from build123d import *

# Parameters (mm, degrees)
F0_R     = 2
F1_DEPTH = 2.5
F2_DEPTH = 4
F3_DEPTH = 8.5
F4_DEPTH = 2
F5_R     = 0.99999


# Not quite as in the source:
# - a fillet or chamfer is up to 0.001 mm smaller than in the source, because OpenCascade refuses the exact size


with BuildPart() as f1:
    # F0 (on Front) → F1 (new body)
    with BuildSketch(Plane.XZ):
        with BuildLine():
            Line((2, 3.4641016151), (2, 0))
            ThreePointArc((2, 0), (0, -2), (-2, 0))
            Line((-2, 0), (-4, 0))
            ThreePointArc((-4, 0), (-2.8284271247, -2.8284271247), (0, -4))
            ThreePointArc((0, -4), (2.8284271247, -2.8284271247), (4, 0))
            ThreePointArc((4, 0), (3.4641016151, 2), (2, 3.4641016151))
        make_face()
        with BuildLine():
            ThreePointArc((0, 4), (1.0352761804, 3.8637033052), (2, 3.4641016151))
            Line((2, 3.4641016151), (2, 4))
            Line((2, 4), (0, 4))
        make_face()
        with BuildLine():
            Line((2, 4), (2, 3.4641016151))
            ThreePointArc((2, 3.4641016151), (3.4641016151, 2), (4, 0))
            ThreePointArc((4, 0), (2.8284271247, -2.8284271247), (0, -4))
            Line((0, -4), (15.6, -4))
            ThreePointArc((15.6, -4), (19.6, 0), (15.6, 4))
            Line((15.6, 4), (2, 4))
        make_face()
        with Locations((15.6, 0)):
            Circle(F0_R, mode=Mode.SUBTRACT)
        with BuildLine():
            ThreePointArc((-2, 0), (0, 2), (2, 0))
            Line((2, 0), (2, 3.4641016151))
            ThreePointArc((2, 3.4641016151), (1.0352761804, 3.8637033052), (0, 4))
            ThreePointArc((0, 4), (-2.8284271247, 2.8284271247), (-4, 0))
            Line((-4, 0), (-2, 0))
        make_face()
        with BuildLine():
            ThreePointArc((-2, 0), (0, -2), (2, 0))
            Line((2, 0), (-2, 0))
        make_face()
        with BuildLine():
            Line((-2, 0), (2, 0))
            ThreePointArc((2, 0), (0, 2), (-2, 0))
        make_face()
    extrude(amount=F1_DEPTH)

    # F0 (on Front) → F2 (join)
    with BuildSketch(Plane.XZ):
        with BuildLine():
            ThreePointArc((-2, 0), (0, 2), (2, 0))
            Line((2, 0), (2, 3.4641016151))
            ThreePointArc((2, 3.4641016151), (1.0352761804, 3.8637033052), (0, 4))
            ThreePointArc((0, 4), (-2.8284271247, 2.8284271247), (-4, 0))
            Line((-4, 0), (-2, 0))
        make_face()
        with BuildLine():
            Line((2, 3.4641016151), (2, 0))
            ThreePointArc((2, 0), (0, -2), (-2, 0))
            Line((-2, 0), (-4, 0))
            ThreePointArc((-4, 0), (-2.8284271247, -2.8284271247), (0, -4))
            ThreePointArc((0, -4), (2.8284271247, -2.8284271247), (4, 0))
            ThreePointArc((4, 0), (3.4641016151, 2), (2, 3.4641016151))
        make_face()
    extrude(amount=-F2_DEPTH)

    # F0 (on Front) → F3 (join)
    with BuildSketch(Plane.XZ):
        with BuildLine():
            ThreePointArc((-2, 0), (0, -2), (2, 0))
            Line((2, 0), (-2, 0))
        make_face()
        with BuildLine():
            Line((-2, 0), (2, 0))
            ThreePointArc((2, 0), (0, 2), (-2, 0))
        make_face()
    extrude(amount=-F3_DEPTH)

    # F0 (on Front) → F4 (join)
    with BuildSketch(Plane.XZ):
        with BuildLine():
            Line((-4, 7.5), (-4, 0))
            ThreePointArc((-4, 0), (-2.8284271247, 2.8284271247), (0, 4))
            Line((0, 4), (2, 4))
            Line((2, 4), (2, 12))
            Line((2, 12), (-4, 12))
            Line((-4, 12), (-4, 10))
            Line((-4, 10), (-1, 10))
            Line((-1, 10), (-1, 7.5))
            Line((-1, 7.5), (-4, 7.5))
        make_face()
        with BuildLine():
            ThreePointArc((0, 4), (1.0352761804, 3.8637033052), (2, 3.4641016151))
            Line((2, 3.4641016151), (2, 4))
            Line((2, 4), (0, 4))
        make_face()
        with BuildLine():
            ThreePointArc((-2, 0), (0, 2), (2, 0))
            Line((2, 0), (2, 3.4641016151))
            ThreePointArc((2, 3.4641016151), (1.0352761804, 3.8637033052), (0, 4))
            ThreePointArc((0, 4), (-2.8284271247, 2.8284271247), (-4, 0))
            Line((-4, 0), (-2, 0))
        make_face()
        with BuildLine():
            ThreePointArc((-2, 0), (0, -2), (2, 0))
            Line((2, 0), (-2, 0))
        make_face()
        with BuildLine():
            Line((-2, 0), (2, 0))
            ThreePointArc((2, 0), (0, 2), (-2, 0))
        make_face()
        with BuildLine():
            Line((2, 3.4641016151), (2, 0))
            ThreePointArc((2, 0), (0, -2), (-2, 0))
            Line((-2, 0), (-4, 0))
            ThreePointArc((-4, 0), (-2.8284271247, -2.8284271247), (0, -4))
            ThreePointArc((0, -4), (2.8284271247, -2.8284271247), (4, 0))
            ThreePointArc((4, 0), (3.4641016151, 2), (2, 3.4641016151))
        make_face()
    extrude(amount=-F4_DEPTH)

    # F5 (radius 1 in the source; OpenCascade refuses exactly that, so slightly less here)
    f5_edges = [f1.edges().sort_by_distance(p)[0] for p in [
        (-1, 0, 8.75),
        (-1, 2, 8.75),
    ]]
    fillet(f5_edges, radius=F5_R)


solid = f1.part
Here's how the part is built. I have some questions about the finished solid (model axes, mm). A direction names the side the tool comes from. Coordinates: 2 decimals unless noted, no trailing zeros. Order: outer loops, then holes, each group sorted by start corner. A loop starts at its lowest first (then second) coordinate and runs counter-clockwise, first axis right, second up.
Item 1: If we section it at B-B on y = -1.25: List the corners of the cut face in (x, z) for me, plus the area to 3 significant figures.
Result sheet:
outline: (0, -4) - (15.6, -4) arc R4 ccw to (15.6, 4) - (0, 4) arc R4 ccw to start; hole circle Ø4 at (15.6, 0)
area: 162 mm2
Item 2: If we section it at D-D on y = 1.25: List the corners of the cut face in (x, z) for me, plus the area to 3 significant figures.
Result sheet:
outline: (-4, 0) arc R4 ccw (long way) to (2, 3.46) - (2, 12) - (-4, 12) - (-4, 10) - (-0.97, 10) - (-0.97, 7.5) - (-4, 7.5) - close
area: 94.5 mm2
Item 3: For faces 5 (the face through (-2, 4, -1)), 6 (the face through (-0.715, 0.301, 8.732)), 7 (the face through (-0.699, 1.715, 8.732)), 8 (the face through (-3.2, 1.4, -2.4)), which set-ups out of +Z, -Z, +X, -X, +Y, -Y let a thin tool reach every point of the face, with its end or its side?
Result sheet:
face 5: +Y
face 6: -X, -Y
face 7: -X, +Y
face 8: none
Item 4: I need wall thicknesses on line 1 (Z direction, x = 15.6, y = -0.85); line 2 (Y direction, x = 5.25, z = 2); line 3 (Y direction, x = -2.25, z = 10.25). Which ranges of each line are inside material? Lowest first, please.
Result sheet:
line 1: z = -4 to -2, 2 to 4
line 2: y = -2.5 to 0
line 3: y = 0 to 2
Item 5: For P1, Ø4.5, axis at x = 15.6, z = 0, coming from the +Y side; P2, Ø0.6, axis at y = 1, z = 7.5, coming from the +X side; P3, Ø5, axis at x = 0.5, z = 7.5, coming from the +Y side; P4, Ø6, axis at x = 9, y = 7, coming from the +Z side, each with a flat end and sliding along its axis, tell me the tip position at first contact or that it passes through.
Result sheet:
P1: stops at y = 0
P2: stops at x = 2
P3: stops at y = 2
P4: passes through
Item 6: If we mould it in two halves opening along Z, with no side actions, what happens to faces 1 (the face through (-2, 1, 7.5)), 2 (the face through (8, -2.5, 0)), 3 (the face through (8, -1, -4)), 4 (the face through (-1, 1, 12))? For each: +Z half, -Z half, draft (parallel to the pull), parting line (faces both ways), or undercut.
Result sheet:
face 1: undercut
face 2: draft
face 3: -Z half
face 4: +Z half
Item 7: If we section it at C-C on x = 16: List the corners of the cut face in (y, z) for me, plus the area to 3 significant figures.
Result sheet:
outline: (-2.5, -3.98) - (0, -3.98) - (0, -1.96) - (-2.5, -1.96) - close; (-2.5, 1.96) - (0, 1.96) - (0, 3.98) - (-2.5, 3.98) - close
area: 10.1 mm2
Item 8: If we section it at A-A on z = -1.5: List the corners of the cut face in (x, y) for me.
Result sheet:
outline: (-3.71, -2.5) - (14.28, -2.5) - (14.28, 0) - (3.71, 0) - (3.71, 4) - (1.32, 4) - (1.32, 8.5) - (-1.32, 8.5) - (-1.32, 4) - (-3.71, 4) - close; (16.92, -2.5) - (19.31, -2.5) - (19.31, 0) - (16.92, 0) - close
